```python
from build123d import *

# Parameters (mm, degrees)
SKETCH1_R           = 10
BOSS_EXTRUDE1_DEPTH = 42
CUT_EXTRUDE1_REACH  = 46.317
SKETCH2_R           = 5.25
SKETCH3_R           = 7.25
CUT_EXTRUDE2_DEPTH  = 32
SKETCH4_R           = 1
SKETCH4_R_2         = 5.25
BOSS_EXTRUDE2_DEPTH = 1.2
CUT_EXTRUDE3_START  = -10
CUT_EXTRUDE3_DEPTH  = 10
DRAFT1_ANGLE        = 1
CHAMFER1_SIZE       = 3
CHAMFER1_SIZE_2     = 3.053760573


with BuildPart() as part:
    # Sketch1 → Boss-Extrude1 (new body)
    with BuildSketch(Plane.XY):
        with Locations(Location((0, 0, 0), (0, 0, 180))):
            Circle(SKETCH1_R)
    extrude(amount=BOSS_EXTRUDE1_DEPTH)

    # Sketch2 → Cut-Extrude1 (cut, up to next)
    with BuildSketch(Plane.XY.offset(42), mode=Mode.PRIVATE) as cut_extrude1_sk1:
        Circle(SKETCH2_R)
    cut_extrude1_tool1 = extrude(cut_extrude1_sk1.sketch, amount=-CUT_EXTRUDE1_REACH, mode=Mode.PRIVATE) & part.part
    add(cut_extrude1_tool1.solids().sort_by_distance((0, 0, 42))[0], mode=Mode.SUBTRACT)

    # Sketch3 → Cut-Extrude2 (cut)
    with BuildSketch(Plane.XY.offset(42)):
        Circle(SKETCH3_R)
    extrude(amount=-CUT_EXTRUDE2_DEPTH, mode=Mode.SUBTRACT)

    # Sketch4 → Boss-Extrude2 (add)
    with BuildSketch(Plane(origin=(0, 0, 0), x_dir=(-1, 0, 0), z_dir=(0, 0, -1))):
        with BuildLine():
            Line((9.98013969, -0.629929975), (11.372178356, -0.629929975))
            ThreePointArc((11.372178356, -0.629929975), (14.722138794, 0.000600368), (11.372121573, 0.630828953))
            Line((11.372121573, 0.630828953), (9.980082907, 0.630828953))
            ThreePointArc((9.980082907, 0.630828953), (-9.99999999, -0.000450385), (9.98013969, -0.629929975))
        make_face()
        with Locations((12.987833992, 0.000522257)):
            Circle(SKETCH4_R, mode=Mode.SUBTRACT)
        with Locations(Location((0, 0, 0), (0, 0, 180))):
            Circle(SKETCH4_R_2, mode=Mode.SUBTRACT)
    extrude(amount=-BOSS_EXTRUDE2_DEPTH)

    # Sketch5 → Cut-Extrude3 (cut)
    with BuildSketch(Plane.XY.offset(42).offset(CUT_EXTRUDE3_START)):
        with BuildLine():
            ThreePointArc((4.358898944, 9), (0, 10), (-4.358898944, 9))
            Line((-4.358898944, 9), (4.358898944, 9))
        make_face()
        with BuildLine():
            Line((4.358898944, -9), (-4.358898944, -9))
            ThreePointArc((-4.358898944, -9), (0, -10), (4.358898944, -9))
        make_face()
    extrude(amount=CUT_EXTRUDE3_DEPTH, mode=Mode.SUBTRACT)

    # Draft1
    draft1_faces = [part.faces().sort_by_distance(p)[0] for p in [
        (-7.25, 0, 26),
    ]]
    draft(draft1_faces, Plane.XY.offset(10), DRAFT1_ANGLE)

    # Chamfer1
    # the kernel refuses this chamfer: 3.053760573, 3 mm, written as the material it adds along each edge
    with BuildSketch(Plane(origin=(0, 0, 10), x_dir=(1, 0, 0), z_dir=(0, -1, 0))) as chamfer1_piece_1_section:
        Polygon((7.25 - CHAMFER1_SIZE, 0), (7.25 + CHAMFER1_SIZE_2 * 0.0174524064385, CHAMFER1_SIZE_2 * 0.999847695226), (7.25, 0), align=None)
    chamfer1_piece_1 = revolve(axis=Axis((0, 0, 10), (0, 0, 1)), mode=Mode.PRIVATE)
    chamfer1_piece_1 = chamfer1_piece_1 - Plane(origin=(0, 0, 12.029896957), x_dir=(1, 0, 0), z_dir=(0, 0, 1)) * Cylinder(5.25, 30, mode=Mode.PRIVATE)
    add(chamfer1_piece_1)


solid = part.part
```
Geometry: final body of the model. Coordinates: model frame, mm. A direction names the side the tool comes from. Round coordinates to 2 decimals unless told otherwise and drop trailing zeros. Order: outer loops, then holes, each group sorted by start corner. A loop starts at its lowest first (then second) coordinate and runs counter-clockwise, first axis right, second up. Notation, with made-up numbers: (12, 2) -> (33, 2) arc R20 cw to (33, 9) -> close; hole circle Ø4 at (87, 3.5). An arc over 180 degrees is marked (long way). Use one line per item in the form item = value.
(1) Section C-C on z = 30. Return loops of the section in (x, y).
Results list:
outline = circle Ø20 at (0, 0); hole circle Ø15.2 at (0, 0)
(2) Ray query, probe 1 along Y at (x, z) = (0, 5.5); probe 2 along X at (y, z) = (-3.25, 23); probe 3 along Y at (x, z) = (-3.25, 28). Return the intervals inside material, ascending. Write a range as [from, to].
Results list:
probe_1 = [-10, -5.25], [5.25, 10]
probe_2 = [-9.46, -6.73], [6.73, 9.46]
probe_3 = [-9.46, -6.83], [6.83, 9.46]
(3) Section B-B on z = 9.5. Return loops of the section in (x, y).
Results list:
outline = circle Ø20 at (0, 0); hole circle Ø10.5 at (0, 0)
(4) Access query for faces 5 (the face through (-0.1, 9.4, 32)), 6 (the face through (-11, 0.631, 1)), 7 (the face through (0, -9, 37)), 8 (the face through (-6, -4.6, 27.7)), 9 (the face through (-11, -0.63, 1)). Directions: +Z, -Z, +X, -X, +Y, -Y. A direction counts if a zero-diameter tool reaches every point of the face in a straight line with its end or side. Return the directions, or none.
Results list:
face_5 = +Z, +X, -X, +Y
face_6 = +Z, -Z, +Y
face_7 = +Z, +X, -X, -Y
face_8 = +Z
face_9 = +Z, -Z, -Y
(5) Draft query along Y for faces 1 (the face through (-9.237, 3.83, 20.706)), 2 (the face through (0, 9, 37)), 3 (the face through (-0.1, -9.4, 32)), 4 (the face through (-11.99, 0.04, 0.59)). Return one class per face: pulls with the +Y half, pulls with the -Y half, needs draft (parallel to the pull), parting line crosses it, or undercut.
Results list:
face_1 = parting line crosses it
face_2 = pulls with the +Y half
face_3 = needs draft
face_4 = undercut
(6) First-contact query: pin 1 Ø4 at (x, y) = (-12.5, -0.5) entering from +Z; pin 2 Ø12 at (x, z) = (-9.5, 25) entering from +Y; pin 3 Ø2.5 at (x, z) = (1, 37.5) entering from -Y; pin 4 Ø9.5 at (x, y) = (0, 0) entering from +Z. Flat tips, straight axial feed; report the tip coordinate or a pass-through.
Results list:
pin_1 = 1.2
pin_2 = 9.37
pin_3 = -9
pin_4 = through
(7) Section A-A on z = 35.5. Return loops of the section in (x, y).
Results list:
outline = (-4.36, -9) -> (4.36, -9) arc R10 ccw to (4.36, 9) -> (-4.36, 9) arc R10 ccw to start; hole circle Ø15.39 at (0, 0)
